Read the model definition and answer for the solid it produces. Units are mm, in the model's axes. A direction names the side the tool comes from. Round coordinates to 2 decimals unless told otherwise and drop trailing zeros. Order: outer loops, then holes, each group sorted by start corner. A loop starts at its lowest first (then second) coordinate and runs counter-clockwise, first axis right, second up. Notation, with made-up numbers: (67, 37) -> (85, 37) arc R29 ccw to (85, 66) -> close; hole circle Ø7 at (6, 6.25). An arc over 180 degrees is marked (long way). Answer as a JSON object with one key per item and string values. Group by question number.
Item 1: Section D-D, the plane z = 7.5 is taken. Count the separate pieces of the cut face and the enclosed holes in it, plus the area to 3 significant figures.
Item 2: Consider probe 1 along X at (y, z) = (-18, 11.5); probe 2 along Y at (x, z) = (21, 6); probe 3 along X at (y, z) = (22, 15). Determine where each line is inside the solid, lowest interval first. Write a range as from..to.
Item 3: Section C-C, the plane y = -46 is taken. Write down the section's boundary in (x, z), plus the area to 3 significant figures.
Item 4: Given P1, Ø3, axis at x = 8.5, y = -11.5, coming from the -Z side; P2, Ø2.5, axis at x = -8.5, z = 2, coming from the -Y side; P3, Ø1.5, axis at x = 34.5, y = -4.5, coming from the +Z side; P4, Ø2.5, axis at y = 42, z = 3, coming from the +X side, each flat-ended and moving along its own axis, determine where each tip first touches the part or whether it passes through.
Item 5: Section A-A, the plane y = 23 is taken. Write down the section's boundary in (x, z).
Item 6: Section B-B, the plane x = 7 is taken. Write down the section's boundary in (y, z).
Item 7: For faces 1 (the flat face through (45, 62, 13)), 2 (the cylindrical face through (19.28, -67.46, 15.49)), 3 (the cylindrical face through (49, -68, 10)), 4 (the flat face through (13.7, -26.3, 3)), 5 (the flat face through (-50, 2, 10)), determine the directions among +Z, -Z, +X, -X, +Y, -Y from which every point of the face is accessible in a straight line to the end or side of a thin tool.
from build123d import *

# Parameters (mm, degrees)
SKETCH_W        = 100
SKETCH_H        = 140
PAD_DEPTH       = 20
SKETCH001_W     = 90
SKETCH001_H     = 135
POCKET_DEPTH    = 15
SKETCH003_R     = 3
POCKET001_DEPTH = 2
SKETCH004_R     = 1.6
POCKET002_DEPTH = 349.411162
SKETCH005_W     = 5
SKETCH005_H     = 50
POCKET003_DEPTH = 20.001
SKETCH006_W     = 30
SKETCH006_H     = 5
POCKET004_DEPTH = 20.001
SKETCH007_W     = 70
SKETCH007_H     = 70.156743
POCKET005_DEPTH = 5.001
SKETCH008_R     = 15
POCKET006_DEPTH = 5.001
FILLET_R        = 5
FILLET001_R     = 5
FILLET002_R     = 15
FILLET003_R     = 15
SKETCH009_R     = 5
PAD001_DEPTH    = 5
SKETCH010_R     = 5
PAD002_DEPTH    = 5
FILLET004_R     = 4.5
FILLET005_R     = 4.5
FILLET006_R     = 4.5
FILLET007_R     = 4.5


with BuildPart() as part:
    # Sketch → Pad (new body)
    with BuildSketch(Plane.XY):
        Rectangle(SKETCH_W, SKETCH_H)
    extrude(amount=PAD_DEPTH)

    # Sketch001 → Pocket (cut)
    with BuildSketch(Plane.XY.offset(20)):
        with Locations((0, 2.5)):
            Rectangle(SKETCH001_W, SKETCH001_H)
    extrude(amount=-POCKET_DEPTH, mode=Mode.SUBTRACT)

    # Sketch003 → Pocket001 (cut)
    with BuildSketch(Plane.XY.offset(5)):
        with Locations((-15, -25)):
            Circle(SKETCH003_R)
    pocket001 = extrude(amount=-POCKET001_DEPTH, mode=Mode.SUBTRACT)

    # Sketch004 → Pocket002 (cut, through all)
    with BuildSketch(Plane.XY.offset(3)):
        with Locations((-15, -25)):
            Circle(SKETCH004_R)
    pocket002 = extrude(amount=-POCKET002_DEPTH, mode=Mode.SUBTRACT)

    # Mirrored: Pocket002, Pocket001 across Sketch004 V_Axis
    add(pocket002.mirror(Plane(origin=(0, 0, 3), x_dir=(0, 0, 1), z_dir=(1, 0, 0))), mode=Mode.SUBTRACT)
    add(pocket001.mirror(Plane(origin=(0, 0, 3), x_dir=(0, 0, 1), z_dir=(1, 0, 0))), mode=Mode.SUBTRACT)

    # Sketch005 → Pocket003 (cut, through all)
    with BuildSketch(Plane.XY.offset(20)):
        with Locations((47.5, 30)):
            Rectangle(SKETCH005_W, SKETCH005_H)
    extrude(amount=-POCKET003_DEPTH, mode=Mode.SUBTRACT)

    # Sketch006 → Pocket004 (cut, through all)
    with BuildSketch(Plane.XY.offset(20)):
        with Locations((0, -67.5)):
            Rectangle(SKETCH006_W, SKETCH006_H)
    extrude(amount=-POCKET004_DEPTH, mode=Mode.SUBTRACT)

    # Sketch007 → Pocket005 (cut, through all)
    with BuildSketch(Plane.XY.offset(5)):
        with Locations((0, 24.921629)):
            Rectangle(SKETCH007_W, SKETCH007_H)
    extrude(amount=-POCKET005_DEPTH, mode=Mode.SUBTRACT)

    # Sketch008 → Pocket006 (cut, through all)
    with BuildSketch(Plane.XY.offset(5)):
        with Locations((0, -65)):
            Circle(SKETCH008_R)
    extrude(amount=-POCKET006_DEPTH, mode=Mode.SUBTRACT)

    # Fillet
    fillet_edges = [part.edges().sort_by_distance(p)[0] for p in [
        (50, -70, 10),
    ]]
    fillet(fillet_edges, radius=FILLET_R)

    # Fillet001
    fillet001_edges = [part.edges().sort_by_distance(p)[0] for p in [
        (-50, -70, 10),
    ]]
    fillet(fillet001_edges, radius=FILLET001_R)

    # Fillet002
    fillet002_edges = [part.edges().sort_by_distance(p)[0] for p in [
        (-15, -67.5, 20),
    ]]
    fillet(fillet002_edges, radius=FILLET002_R)

    # Fillet003
    fillet003_edges = [part.edges().sort_by_distance(p)[0] for p in [
        (15, -67.5, 20),
    ]]
    fillet(fillet003_edges, radius=FILLET003_R)

    # Sketch009 → Pad001 (new body)
    with BuildSketch(Plane.XY.offset(5)):
        with Locations((35, 64.8)):
            Circle(SKETCH009_R)
    pad001 = extrude(amount=PAD001_DEPTH)

    # Mirrored001: Pad001 across Sketch009 V_Axis
    add(pad001.mirror(Plane(origin=(0, 0, 5), x_dir=(0, 0, 1), z_dir=(1, 0, 0))))

    # Sketch010 → Pad002 (new body)
    with BuildSketch(Plane.XY.offset(5)):
        with Locations((-35, -55)):
            Circle(SKETCH010_R)
    pad002 = extrude(amount=PAD002_DEPTH)

    # Mirrored002: Pad002 across Sketch010 V_Axis
    add(pad002.mirror(Plane(origin=(0, 0, 5), x_dir=(0, 0, 1), z_dir=(1, 0, 0))))

    # Fillet004
    fillet004_edges = [part.edges().sort_by_distance(p)[0] for p in [
        (-40, -55, 10),
    ]]
    fillet(fillet004_edges, radius=FILLET004_R)

    # Fillet005
    fillet005_edges = [part.edges().sort_by_distance(p)[0] for p in [
        (40, -55, 10),
    ]]
    fillet(fillet005_edges, radius=FILLET005_R)

    # Fillet006
    fillet006_edges = [part.edges().sort_by_distance(p)[0] for p in [
        (30, 64.8, 10),
    ]]
    fillet(fillet006_edges, radius=FILLET006_R)

    # Fillet007
    fillet007_edges = [part.edges().sort_by_distance(p)[0] for p in [
        (-30, 64.8, 10),
    ]]
    fillet(fillet007_edges, radius=FILLET007_R)


solid = part.part
Values found:
{
 "1": {"separate pieces": "7", "enclosed holes": "0", "area": "1,700 mm2"},
 "2": {"probe 1": "-50..-45, 45..50", "probe 2": "-70..-65", "probe 3": "-50..-45"},
 "3": {"outline": "(-50, 0) -> (50, 0) -> (50, 20) -> (45, 20) -> (45, 5) -> (-45, 5) -> (-45, 20) -> (-50, 20) -> close", "area": "650 mm2"},
 "4": {"P1": "z = 0", "P2": "y = -53.6", "P3": "z = 5", "P4": "x = 45"},
 "5": {"outline": "(-50, 0) -> (-35, 0) -> (-35, 5) -> (-45, 5) -> (-45, 20) -> (-50, 20) -> close; (35, 0) -> (45, 0) -> (45, 5) -> (35, 5) -> close"},
 "6": {"outline": "(-51.73, 0) -> (-10.16, 0) -> (-10.16, 5) -> (-51.73, 5) -> close; (60, 0) -> (70, 0) -> (70, 5) -> (60, 5) -> close"},
 "7": {"face 1": "+Z, +Y", "face 2": "+Z, +Y, -Y", "face 3": "+Z, -Z, +X, -Y", "face 4": "+Z", "face 5": "+Z, -Z, -X, +Y, -Y"}
}
